Geometry: final body of the model. Coordinates: model frame, mm. Round coordinates to 2 decimals unless told otherwise and drop trailing zeros. Loops run counter-clockwise (first coordinate to the right, second up) from the corner with the lowest first, then second, coordinate; pieces in that order, holes last. Notation, with made-up numbers: (-27.5, -39) - (17.5, -39) arc R22 cw to (17.5, -14) - close; hole circle Ø3 at (-35.75, 35). An arc over 180 degrees is marked (long way). Return JSON: item names as keys, results as strings. Group by question number.
1. Section B-B on z = 57. Return loops of the section in (x, y), and give its area (3 significant figures).
2. Section A-A on y = 0. Count the separate pieces of the cut face and the enclosed holes in it, and give its area (3 significant figures).
3. Material intervals for probe 1 along Z at (x, y) = (-1.5, 0); probe 2 along Y at (x, z) = (0, 41.5); probe 3 along Y at (x, z) = (-0.75, 41.5), sorted ascending.
4. First-contact query: pin 1 Ø1 at (y, z) = (-1.5, 173) entering from -X; pin 2 Ø1 at (y, z) = (0.5, 2.5) entering from -X; pin 3 Ø2.5 at (y, z) = (-0.5, 4) entering from +X; pin 4 Ø1.8 at (y, z) = (0, 41.5) entering from +X. Flat tips, straight axial feed; report the tip coordinate or a pass-through.
5. Draft query along Z for faces 1 (the face through (0, 0, 275)), 2 (the face through (0, 0, 0)). Return one class per face: +Z half, -Z half, draft (parallel to the pull), parting line (faces both ways), or undercut.
from build123d import *

# Parameters (mm, degrees)
SKETCH1_R                       = 3
BOSS_EXTRUDE1_DEPTH             = 275
SKETCH3_W                       = 0.8
SKETCH3_H                       = 0.5
CUT_EXTRUDE2_DEPTH              = 276.032725326
CUT_EXTRUDE2_DEPTH_BACK         = 276.032725326
SKETCH4_W                       = 3.470061058
SKETCH4_H                       = 7
SKETCH4_W_2                     = 2.92528695
CHAMFER1_SIZE                   = 0.3
RETAINING_GROOVES_D5P7_1_START  = 7.05
SKETCH5_R                       = 2.85
SKETCH5_R_2                     = 2.49
RETAINING_GROOVES_D5P7_1_DEPTH  = 0.8
RETAINING_GROOVES_D5P7_2_START  = 13
SKETCH6_R                       = 2.85
SKETCH6_R_2                     = 2.49
RETAINING_GROOVES_D5P7_2_DEPTH  = 0.8
RETAINING_GROOVES_D5P7_3_START  = 260.25
SKETCH7_R                       = 2.85
SKETCH7_R_2                     = 2.49
RETAINING_GROOVES_D5P7_3_DEPTH  = 0.8
RETAINING_GROOVES_D5P7_4_START  = 266.2
SKETCH8_R                       = 2.85
SKETCH8_R_2                     = 2.49
RETAINING_GROOVES_D5P7_4_DEPTH  = 0.8
TWO_HUB_CROSS_PIN_D2_DEPTH      = 276.032725326
TWO_HUB_CROSS_PIN_D2_DEPTH_BACK = 276.032725326
SKETCH9_R                       = 1


with BuildPart() as part:
    # Sketch1 → Boss-Extrude1 (new body)
    with BuildSketch(Plane.XY):
        Circle(SKETCH1_R)
    extrude(amount=BOSS_EXTRUDE1_DEPTH)

    # Sketch3 → Cut-Revolve1 (revolve, cut)
    with BuildSketch(Plane(origin=(0, 0, 0), x_dir=(0, 0, -1), z_dir=(1, 0, 0)), mode=Mode.PRIVATE) as cut_revolve1_sk:
        with Locations((-266.6, 2.75)):
            Rectangle(SKETCH3_W, SKETCH3_H)
        with Locations((-260.65, 2.75)):
            Rectangle(SKETCH3_W, SKETCH3_H)
        with Locations((-13.4, 2.75)):
            Rectangle(SKETCH3_W, SKETCH3_H)
        with Locations((-7.45, 2.75)):
            Rectangle(SKETCH3_W, SKETCH3_H)
    revolve(cut_revolve1_sk.sketch.rotate(Axis((0, 0, 263.365004794), (0, 0, -1)), 90), axis=Axis((0, 0, 263.365004794), (0, 0, -1)), mode=Mode.SUBTRACT)

    # Sketch4 → Cut-Extrude2 (cut, two sides: drawn at the far end of the back side and taken through both)
    with BuildSketch(Plane(origin=(0, 0, 0), x_dir=(1, 0, 0), z_dir=(0, 1, 0)).offset(-CUT_EXTRUDE2_DEPTH_BACK)):
        with Locations((4.235030529, -3.5)):
            Rectangle(SKETCH4_W, SKETCH4_H)
        with Locations((-3.962643475, -3.5)):
            Rectangle(SKETCH4_W_2, SKETCH4_H)
    extrude(amount=CUT_EXTRUDE2_DEPTH + CUT_EXTRUDE2_DEPTH_BACK, mode=Mode.SUBTRACT)

    # Chamfer1
    chamfer1_edges = [part.edges().sort_by_distance(p)[0] for p in [
        (0, 3, 0),
        (0, -3, 0),
    ]]
    chamfer(chamfer1_edges, length=CHAMFER1_SIZE)

    # Sketch5 → Retaining_Grooves_D5p7_1 (add)
    with BuildSketch(Plane.XY.offset(RETAINING_GROOVES_D5P7_1_START)):
        Circle(SKETCH5_R)
        Circle(SKETCH5_R_2, mode=Mode.SUBTRACT)
    extrude(amount=RETAINING_GROOVES_D5P7_1_DEPTH)

    # Sketch6 → Retaining_Grooves_D5p7_2 (add)
    with BuildSketch(Plane.XY.offset(RETAINING_GROOVES_D5P7_2_START)):
        Circle(SKETCH6_R)
        Circle(SKETCH6_R_2, mode=Mode.SUBTRACT)
    extrude(amount=RETAINING_GROOVES_D5P7_2_DEPTH)

    # Sketch7 → Retaining_Grooves_D5p7_3 (add)
    with BuildSketch(Plane.XY.offset(RETAINING_GROOVES_D5P7_3_START)):
        Circle(SKETCH7_R)
        Circle(SKETCH7_R_2, mode=Mode.SUBTRACT)
    extrude(amount=RETAINING_GROOVES_D5P7_3_DEPTH)

    # Sketch8 → Retaining_Grooves_D5p7_4 (add)
    with BuildSketch(Plane.XY.offset(RETAINING_GROOVES_D5P7_4_START)):
        Circle(SKETCH8_R)
        Circle(SKETCH8_R_2, mode=Mode.SUBTRACT)
    extrude(amount=RETAINING_GROOVES_D5P7_4_DEPTH)

    # Sketch9 → Two_Hub_Cross_Pin_D2 (cut, two sides: drawn at the far end of the back side and taken through both)
    with BuildSketch(Plane(origin=(0, 0, 0), x_dir=(0, 0, -1), z_dir=(1, 0, 0)).offset(-TWO_HUB_CROSS_PIN_D2_DEPTH_BACK)):
        with Locations((-41.5, 0)):
            Circle(SKETCH9_R)
        with Locations((-243.5, 0)):
            Circle(SKETCH9_R)
    extrude(amount=TWO_HUB_CROSS_PIN_D2_DEPTH + TWO_HUB_CROSS_PIN_D2_DEPTH_BACK, mode=Mode.SUBTRACT)


solid = part.part
Taken from the geometry:
{
 "1": {"outline": "circle Ø6 at (0, 0)", "area": "28.3 mm2"},
 "2": {"separate pieces": "3", "enclosed holes": "0", "area": "1,620 mm2"},
 "3": {"probe 1": "0 to 40.5, 42.5 to 242.5, 244.5 to 275", "probe 2": "-3 to -1, 1 to 3", "probe 3": "-2.9 to -1, 1 to 2.9"},
 "4": {"pin 1": "x = -2.83", "pin 2": "x = -2.5", "pin 3": "x = 2.5", "pin 4": "through"},
 "5": {"face 1": "+Z half", "face 2": "-Z half"}
}
